```python
from build123d import *

# Parameters (mm, degrees)
F0_W     = 1380
F0_H     = 60
F1_DEPTH = 3
F2_W     = 1380
F2_H     = 10
F3_DEPTH = 1.5
F4_R     = 2
F5_W     = 145
F5_H     = 35
F6_DEPTH = 3
F8_DEPTH = 1.5


with BuildPart() as f1:
    # F0 (on Front) → F1 (new body)
    with BuildSketch(Plane.XZ):
        Rectangle(F0_W, F0_H)
    extrude(amount=F1_DEPTH)

    # F2 (on face) → F3 (cut)
    with BuildSketch(Plane(origin=(0, 0, 0), x_dir=(-1, 0, 0), z_dir=(0, 1, 0))):
        with Locations((0, -25)):
            Rectangle(F2_W, F2_H)
    extrude(amount=-F3_DEPTH, mode=Mode.SUBTRACT)

    # F4
    f4_edges = [f1.edges().sort_by_distance(p)[0] for p in [
        (690, -2.25, -30),
        (690, -1.5, 30),
        (-690, -1.5, 30),
        (-690, -2.25, -30),
    ]]
    fillet(f4_edges, radius=F4_R)

    # F5 (on face) → F6 (cut)
    with BuildSketch(Plane.XZ.offset(3)):
        with Locations((-597.5, 12.5)):
            Rectangle(F5_W, F5_H)
    extrude(amount=-F6_DEPTH, mode=Mode.SUBTRACT)

    # F7 (on face) → F8 (cut)
    with BuildSketch(Plane(origin=(0, 0, 0), x_dir=(-1, 0, 0), z_dir=(0, 1, 0))):
        Polygon((525, -5), (525, 30), (521, 30), (521, -9), (674, -9), (674, 30), (670, 30), (670, -5), align=None)
    extrude(amount=-F8_DEPTH, mode=Mode.SUBTRACT)


solid = f1.part
```
Input: part model. Units: mm. Frame: model coordinates. Round coordinates to 2 decimals unless told otherwise and drop trailing zeros. Write each loop counter-clockwise with the first axis right and the second up, starting at its lowest first coordinate (ties: lowest second). Pieces come first, ordered by that corner, then holes. Notation, with made-up numbers: M 53,33 L 81,33 A26 cw 81,54 Z; hole C -7.5,-2.5 d9. An arc over 180 degrees is marked long. Write each question's results on one line, items separated by ' | '.
Q1. Draft query along X for faces 1 (the face through (-597, -1.5, -7)), 2 (the face through (-10, -3, 0)). Return one class per face: released by +X, released by -X, zero draft, split by the parting line, or undercut.
Results:
face 1: undercut | face 2: zero draft
Q2. Section query B-B (y = -2.3). Return loops of the section in (x, z), and give its area (3 significant figures).
Results:
outline: M -690,-28 A2 ccw -688,-30 L 688,-30 A2 ccw 690,-28 L 690,28 A2 ccw 688,30 L -525,30 L -525,-5 L -670,-5 L -670,30 L -688,30 A2 ccw -690,28 Z | area: 77,700 mm^2
Q3. Pin query (flat end, axial travel): P1, Ø3, axis at x = -176.5, z = -26, coming from the +Y side; P2, Ø1.6, axis at x = 93, y = -1, coming from the -Z side; P3, Ø1.2, axis at x = -584.5, y = -1, coming from the +Z side. Return the tip coordinate at first contact, or that it passes through.
Results:
P1: stops at y = -1.5 | P2: stops at z = -30 | P3: stops at z = -5
Q4. Section query C-C (x = 589.5). Return loops of the section in (y, z), and give its area (3 significant figures).
Results:
outline: M -3,-30 L -1.5,-30 L -1.5,-20 L 0,-20 L 0,30 L -3,30 Z | area: 165 mm^2
Q5. Line query: line 1 along X through (y, z) = (-1.4, 16.5); line 2 along X through (y, z) = (-2.7, 16.5); line 3 along Z through (x, y) = (-562, -2.15). Output: solid intervals per line, ascending.
Results:
line 1: x = -690 to -674, -521 to 690 | line 2: x = -690 to -670, -525 to 690 | line 3: z = -30 to -5
Q6. Section query A-A (z = 17). Return loops of the section in (x, y), and give its area (3 significant figures).
Results:
outline: M -690,-3 L -670,-3 L -670,-1.5 L -674,-1.5 L -674,0 L -690,0 Z; M -525,-3 L 690,-3 L 690,0 L -521,0 L -521,-1.5 L -525,-1.5 Z | area: 3,690 mm^2
